For this review, take the finished solid that the model builds, in its own axes (mm). A direction names the side the tool comes from. Round coordinates to 2 decimals unless told otherwise and drop trailing zeros. Write each loop counter-clockwise with the first axis right and the second up, starting at its lowest first coordinate (ties: lowest second). Pieces come first, ordered by that corner, then holes. Notation, with made-up numbers: M 79,84.25 L 102,84.25 A20 cw 102,104.25 Z; hole C -39,78.5 d3. An arc over 180 degrees is marked long. One line per question, with ' | ' between items.
```python
from build123d import *

# Parameters (mm, degrees)
SKETCH_1_W          = 70
SKETCH_1_H          = 100
SKETCH_1_R          = 1.6
EXTRUDE_1_DEPTH     = 4
SKETCH_2_W          = 25
SKETCH_2_H          = 3
SKETCH_2_W_2        = 15
EXTRUDE_2_DEPTH     = 82
SKETCH_3_R          = 1.55
SKETCH_3_R_2        = 1.539226355
CUT_EXTRUDE_1_DEPTH = 8
EXTRUDE_3_DEPTH     = 2
SKETCH_7_R          = 1.6
EXTRUDE_5_DEPTH     = 82
SKETCH_10_R         = 1.55
CUT_EXTRUDE_2_DEPTH = 118.749734607


with BuildPart() as part:
    # 草图1 → 凸台-拉伸1 (new body)
    with BuildSketch(Plane.XY):
        with Locations((3.334002404, 0)):
            Rectangle(SKETCH_1_W, SKETCH_1_H)
        with Locations((34.334002404, 26.5)):
            Circle(SKETCH_1_R, mode=Mode.SUBTRACT)
        with Locations((-16.665997596, -46)):
            Circle(SKETCH_1_R, mode=Mode.SUBTRACT)
        with Locations((3.334002404, 46)):
            Circle(SKETCH_1_R, mode=Mode.SUBTRACT)
        with Locations((10.834002404, 28.5)):
            Circle(SKETCH_1_R, mode=Mode.SUBTRACT)
        with Locations((10.834002404, -2.5)):
            Circle(SKETCH_1_R, mode=Mode.SUBTRACT)
        with Locations((34.334002404, -11.5)):
            Circle(SKETCH_1_R, mode=Mode.SUBTRACT)
        with Locations(Location((-27.665997596, 26.5, 0), (0, 0, 180))):
            Circle(SKETCH_1_R, mode=Mode.SUBTRACT)
        with Locations(Location((-4.165997596, 28.5, 0), (0, 0, 180))):
            Circle(SKETCH_1_R, mode=Mode.SUBTRACT)
        with Locations(Location((-4.165997596, -2.5, 0), (0, 0, 180))):
            Circle(SKETCH_1_R, mode=Mode.SUBTRACT)
        with Locations(Location((-27.665997596, -11.5, 0), (0, 0, 180))):
            Circle(SKETCH_1_R, mode=Mode.SUBTRACT)
        with Locations(Location((23.334002404, -46, 0), (0, 0, 180))):
            Circle(SKETCH_1_R, mode=Mode.SUBTRACT)
    extrude(amount=EXTRUDE_1_DEPTH)

    # 草图2 → 凸台-拉伸2 (add)
    with BuildSketch(Plane.XY.offset(4)):
        with Locations((-9.165997596, -19.5)):
            Rectangle(SKETCH_2_W, SKETCH_2_H)
        with Locations((10.834002404, -19.5)):
            Rectangle(SKETCH_2_W_2, SKETCH_2_H)
    extrude(amount=EXTRUDE_2_DEPTH)

    # 草图3 → 切除-拉伸1 (cut)
    with BuildSketch(Plane.XZ.offset(21)):
        with Locations(Location((-18.665997596, 83, 0), (0, 0, 270))):
            Circle(SKETCH_3_R)
        with Locations(Location((10.334002404, 83, 0), (0, 0, 270))):
            Circle(SKETCH_3_R)
        with Locations(Location((-1.685541592, 63, 0), (0, 0, 270))):
            Circle(SKETCH_3_R)
        with Locations(Location((-1.685541592, 56, 0), (0, 0, 270))):
            Circle(SKETCH_3_R_2)
        with Locations(Location((-8.685541592, 56, 0), (0, 0, 270))):
            Circle(SKETCH_3_R)
        with Locations(Location((-1.685541592, 49, 0), (0, 0, 270))):
            Circle(SKETCH_3_R)
        with Locations(Location((5.314458408, 56, 0), (0, 0, 270))):
            Circle(SKETCH_3_R)
        with Locations(Location((-18.665997596, 29, 0), (0, 0, 270))):
            Circle(SKETCH_3_R)
        with Locations(Location((10.334002404, 29, 0), (0, 0, 270))):
            Circle(SKETCH_3_R)
    extrude(amount=-CUT_EXTRUDE_1_DEPTH, mode=Mode.SUBTRACT)

    # 草图6 → 凸台-拉伸3 (add, symmetric)
    with BuildSketch(Plane.YZ.offset(-1.665997596)):
        Polygon((-21, 44.617390455), (-21, 4), (-35.87334108, 4), align=None)
    extrude(amount=EXTRUDE_3_DEPTH, both=True)

    # 草图7 → 凸台-拉伸5 (add)
    with BuildSketch(Plane.XY.offset(4)):
        with Locations(Location((-27.665997596, -11.5, 0), (0, 0, 180))):
            Circle(SKETCH_7_R)
        Polygon((-24.665997596, 9), (-24.665997596, -21), (-21.665997596, -21), (-21.665997596, -18), (-21.665997596, 9), align=None)
    extrude(amount=EXTRUDE_5_DEPTH)


with BuildPart() as extrude_5_kept_piece:
    # of the separate pieces the step leaves, the one the design keeps (extrude_5_pieces_kept)
    add(part.part.solids().sort_by_distance((-31.665997596, 50, 0))[0])

    # 草图10 → 切除-拉伸2 (cut, through all)
    with BuildSketch(Plane(origin=(-24.665997596, 0, 0), x_dir=(0, 0, -1), z_dir=(1, 0, 0))):
        with Locations(Location((-75, 6, 0), (0, 0, 270))):
            Circle(SKETCH_10_R)
        with Locations(Location((-75, -12, 0), (0, 0, 180))):
            Circle(SKETCH_10_R)
        with Locations(Location((-56, -3, 0), (0, 0, 180))):
            Circle(SKETCH_10_R)
        with Locations(Location((-37, 6, 0), (0, 0, 180))):
            Circle(SKETCH_10_R)
        with Locations(Location((-37, -12, 0), (0, 0, 270))):
            Circle(SKETCH_10_R)
    extrude(amount=CUT_EXTRUDE_2_DEPTH, mode=Mode.SUBTRACT)


solid = extrude_5_kept_piece.part
```
Item 1: Take a section at C-C (x = 14). Write out the cut boundary in (y, z).
Results:
outline: M -50,0 L 50,0 L 50,4 L -18,4 L -18,86 L -21,86 L -21,4 L -50,4 Z
Item 2: Mouldability with a two-part tool opening along Z and no side actions: class faces 4 (the face through (18.334, -20, 44)), 5 (the face through (-11.2, -18.2, 86)), 6 (the face through (-23.187, 5.534, 38.478)) as +Z half, -Z half, draft (parallel to the pull), parting line (faces both ways), or undercut.
Results:
face 4: draft | face 5: +Z half | face 6: undercut
Item 3: To check wall thickness, follow line 1 along Y through (x, z) = (-22.25, 75); line 2 along X through (y, z) = (-20, 56); line 3 along Z through (x, y) = (-22.7, -3). State the ranges of each line that lie inside material, in increasing order. Write a range as from..to.
Results:
line 1: -21..-13.55, -10.45..4.45, 7.55..9 | line 2: -24.67..-10.24, -7.14..-3.22, -0.15..3.76, 6.86..18.33 | line 3: 0..54.45, 57.55..86
Item 4: Machinability: for faces 1 (the face through (-21.666, -5, 44)), 2 (the face through (5.78, -19.52, 54.52)), 3 (the face through (-8, -21, 44)), which of the approach directions +Z, -Z, +X, -X, +Y, -Y give a long, thin tool a straight path to every point of the face, cutting with its end or side? Answer none if there is none.
Results:
face 1: +Z, +X, +Y | face 2: +Y, -Y | face 3: +Z, -Y
Item 5: Take a section at D-D (z = 56). Write out the cut boundary in (x, y).
Results:
outline: M -24.67,-21 L -10.24,-21 L -10.24,-18 L -21.67,-18 L -21.67,-4.55 L -24.67,-4.55 Z; M -24.67,-1.45 L -21.67,-1.45 L -21.67,9 L -24.67,9 Z; M -7.14,-21 L -3.22,-21 L -3.22,-18 L -7.14,-18 Z; M -0.15,-21 L 3.76,-21 L 3.76,-18 L -0.15,-18 Z; M 6.86,-21 L 18.33,-21 L 18.33,-18 L 6.86,-18 Z
Item 6: Take a section at B-B (z = 75). Write out the cut boundary in (x, y), then the cut area to 3 significant figures.
Results:
outline: M -24.67,-21 L 18.33,-21 L 18.33,-18 L -21.67,-18 L -21.67,-13.55 L -24.67,-13.55 Z; M -24.67,-10.45 L -21.67,-10.45 L -21.67,4.45 L -24.67,4.45 Z; M -24.67,7.55 L -21.67,7.55 L -21.67,9 L -24.67,9 Z | area: 191 mm2
Item 7: Insertion check: pin 1 Ø12 at (y, z) = (-28, 18.5) entering from -X; pin 2 Ø8 at (x, z) = (4.5, 64.5) entering from +Y; pin 3 Ø4 at (x, y) = (-27.67, -11.5) entering from -Z; pin 4 Ø1.9 at (x, y) = (3.33, 46) entering from -Z. Each pin has a flat end and moves straight along its axis. Give the tip position at first contact, or say it passes through.
Results:
pin 1: x = -3.67 | pin 2: y = -18 | pin 3: z = 0 | pin 4: through
Item 8: Take a section at A-A (y = 6). Write out the cut boundary in (x, z).
Results:
outline: M -31.67,0 L 38.33,0 L 38.33,4 L -21.67,4 L -21.67,35.45 L -24.67,35.45 L -24.67,4 L -31.67,4 Z; M -24.67,38.55 L -21.67,38.55 L -21.67,73.45 L -24.67,73.45 Z; M -24.67,76.55 L -21.67,76.55 L -21.67,86 L -24.67,86 Z
